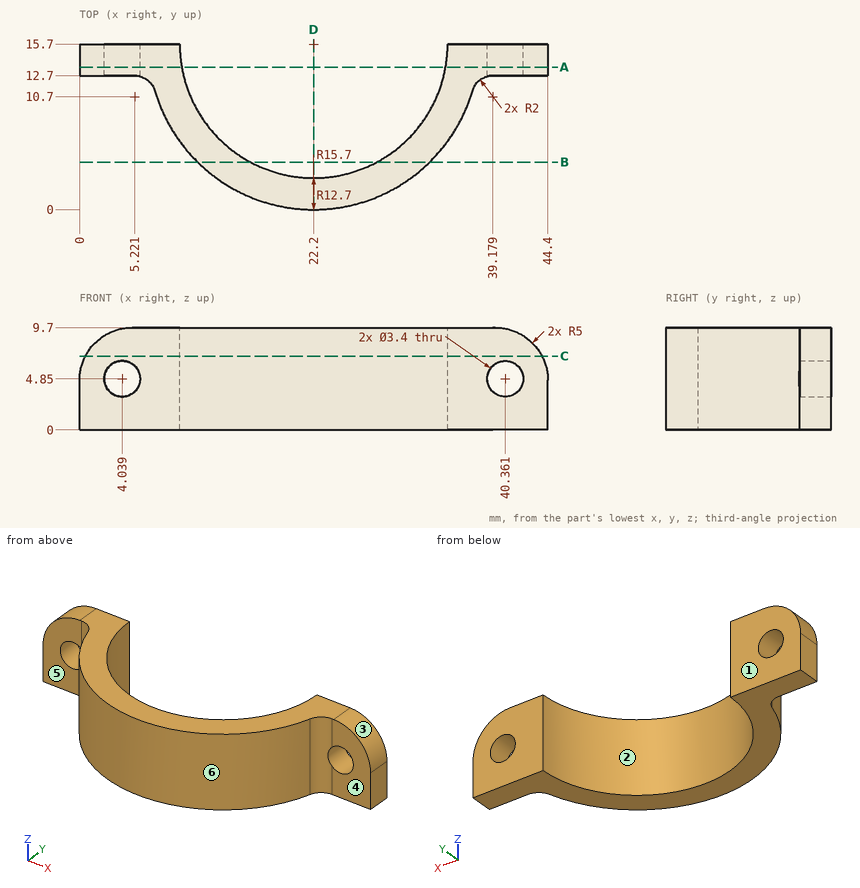
Study the drawing (mm; zero at the part's minimum x, y, z) and answer. A direction names the side the tool comes from. Round coordinates to 2 decimals unless told otherwise and drop trailing zeros. Write each loop counter-clockwise with the first axis right and the second up, starting at its lowest first coordinate (ties: lowest second). Pieces come first, ordered by that corner, then holes.
1) A cutting plane is placed at B-B (y = 4.5). Give the vertices of the cut face in (x, z), plus the area to 3 significant figures.
2) A cutting plane is placed at C-C (z = 7). Give the vertices of the cut face in (x, y) (1 decimal), plus the area to 3 significant figures.
3) A cutting plane is placed at A-A (y = 13.5). Give the vertices of the cut face in (x, z), plus the area to 3 significant figures.
4) A cutting plane is placed at D-D (x = 22.2). Give the vertices of the cut face in (y, z), plus the area to 3 significant figures.
5) A tool of negligible diameter and unlimited length cuts with its end or side. For the marked faces 4, 5 and 6, from which of +Z, -Z, +X, -X, +Y, -Y can it reach the whole face along a straight path? Write none if from no direction.
6) The mould has two halves that part along X. Classify the marked faces 1, 2 and 3: pulls with the +X half, pulls with the -X half, needs draft (parallel to the pull), parting line crosses it, or undercut.
7) Given pin 1 Ø1.5 at (y, z) = (6, 4.5) entering from -X; pin 2 Ø4 at (x, z) = (29, 3) entering from +Y; pin 3 Ø2.5 at (x, z) = (41, 5.5) entering from -Y; pin 4 Ø4 at (x, z) = (40.36, 4.85) entering from +Y, each flat-ended and moving along its own axis, determine where each tip first touches the part or whether it passes through.
8) Straight lines are drawn through the part: line 1 (X direction, y = 13.3, z = 4.85); line 2 (X direction, y = 14, z = 4.85) (1 decimal); line 3 (X direction, y = 4.5, z = 4.5) (1 decimal). For each, find the intervals that lie inside material, in ascending order.
Completed:
1. outline: (11.2, 0) - (16.21, 0) - (16.21, 9.7) - (11.2, 9.7) - close; (28.19, 0) - (33.2, 0) - (33.2, 9.7) - (28.19, 9.7) - close
1. area: 97.3 mm2
2. outline: (0.6, 12.7) - (5.2, 12.7) arc R2 cw to (7.1, 11.3) arc R15.7 ccw to (37.3, 11.3) arc R2 cw to (39.2, 12.7) - (43.8, 12.7) - (43.8, 15.7) - (34.9, 15.7) arc R12.7 cw to (9.5, 15.7) - (0.6, 15.7) - close
2. area: 171 mm2
3. outline: (0, 0) - (9.69, 0) - (9.69, 9.7) - (5, 9.7) arc R5 ccw to (0, 4.7) - close; (34.71, 0) - (44.4, 0) - (44.4, 4.7) arc R5 ccw to (39.4, 9.7) - (34.71, 9.7) - close; hole circle Ø3.4 at (4.04, 4.85); hole circle Ø3.4 at (40.36, 4.85)
3. area: 159 mm2
4. outline: (0, 0) - (3, 0) - (3, 9.7) - (0, 9.7) - close
4. area: 29.1 mm2
5. face 4: +Z, -Z, +X, -Y
5. face 5: +Z, -Z, -X, -Y
5. face 6: +Z, -Z, -Y
6. face 1: needs draft
6. face 2: undercut
6. face 3: pulls with the +X half
7. pin 1: stops at x = 9.3
7. pin 2: stops at y = 6.54
7. pin 3: stops at y = 12.7
7. pin 4: stops at y = 15.7
8. line 1: x = 0 to 2.34, 5.74 to 9.73, 34.67 to 38.66, 42.06 to 44.4
8. line 2: x = 0 to 2.3, 5.7 to 9.6, 34.8 to 38.7, 42.1 to 44.4
8. line 3: x = 11.2 to 16.2, 28.2 to 33.2
